Source: CAD feature listing. Evaluate the final solid. Frame: model axes, mm. Coordinates: 2 decimals unless noted, no trailing zeros. Order: outer loops, then holes, each group sorted by start corner. A loop starts at its lowest first (then second) coordinate and runs counter-clockwise, first axis right, second up. Notation, with made-up numbers: (-24, 0) - (15, 0) arc R26 ccw to (15, 26) - close; hole circle Ø6 at (49, -36.75). An arc over 180 degrees is marked (long way). One line per question, with ' | ' between items.
from build123d import *

# Parameters (mm, degrees)
F0_R     = 57.15
F0_R_2   = 9.525
F1_DEPTH = 3.175


with BuildPart() as f1:
    # F0 (on Front) → F1 (new body, symmetric)
    with BuildSketch(Plane.XZ):
        Circle(F0_R)
        with BuildLine():
            ThreePointArc((-32.267608, -44.82798), (-36.315903, -39.658594), (-31.489624, -35.206824))
            ThreePointArc((-31.489624, -35.206824), (-31.099362, -35.222577), (-30.711639, -35.269733))
            ThreePointArc((-30.711639, -35.269733), (-10.931764, -30.012682), (1.53061, -13.777866))
            ThreePointArc((1.53061, -13.777866), (1.553959, -13.706546), (1.578414, -13.635598))
            ThreePointArc((1.578414, -13.635598), (7.66651, -10.668663), (10.727742, -16.709895))
            ThreePointArc((10.727742, -16.709895), (10.704393, -16.781215), (10.679938, -16.852163))
            ThreePointArc((10.679938, -16.852163), (-5.618196, -38.070526), (-31.489624, -44.890889))
            ThreePointArc((-31.489624, -44.890889), (-31.879886, -44.875136), (-32.267608, -44.82798))
        make_face(mode=Mode.SUBTRACT)
        with BuildLine():
            ThreePointArc((-54.514813, -8.881524), (-53.722082, -2.36364), (-47.16151, -2.628457))
            ThreePointArc((-47.16151, -2.628457), (-46.896692, -2.915553), (-46.655876, -3.223059))
            ThreePointArc((-46.655876, -3.223059), (-28.952096, -13.492246), (-8.660118, -10.824727))
            ThreePointArc((-8.660118, -10.824727), (-8.593177, -10.790807), (-8.525717, -10.757931))
            ThreePointArc((-8.525717, -10.757931), (-2.122843, -12.964926), (-4.230021, -19.401339))
            ThreePointArc((-4.230021, -19.401339), (-4.296962, -19.43526), (-4.364422, -19.468135))
            ThreePointArc((-4.364422, -19.468135), (-30.892592, -22.947263), (-54.009178, -9.476126))
            ThreePointArc((-54.009178, -9.476126), (-54.273996, -9.18903), (-54.514813, -8.881524))
        make_face(mode=Mode.SUBTRACT)
        with BuildLine():
            ThreePointArc((8.881524, -54.514813), (2.36364, -53.722082), (2.628457, -47.16151))
            ThreePointArc((2.628457, -47.16151), (2.915553, -46.896692), (3.223059, -46.655876))
            ThreePointArc((3.223059, -46.655876), (13.492246, -28.952096), (10.824727, -8.660118))
            ThreePointArc((10.824727, -8.660118), (10.790807, -8.593177), (10.757931, -8.525717))
            ThreePointArc((10.757931, -8.525717), (12.964926, -2.122843), (19.401339, -4.230021))
            ThreePointArc((19.401339, -4.230021), (19.43526, -4.296962), (19.468135, -4.364422))
            ThreePointArc((19.468135, -4.364422), (22.947263, -30.892592), (9.476126, -54.009178))
            ThreePointArc((9.476126, -54.009178), (9.18903, -54.273996), (8.881524, -54.514813))
        make_face(mode=Mode.SUBTRACT)
        with BuildLine():
            ThreePointArc((44.82798, -32.267608), (39.658594, -36.315903), (35.206824, -31.489624))
            ThreePointArc((35.206824, -31.489624), (35.222577, -31.099362), (35.269733, -30.711639))
            ThreePointArc((35.269733, -30.711639), (30.012682, -10.931764), (13.777866, 1.53061))
            ThreePointArc((13.777866, 1.53061), (13.706546, 1.553959), (13.635598, 1.578414))
            ThreePointArc((13.635598, 1.578414), (10.668663, 7.66651), (16.709895, 10.727742))
            ThreePointArc((16.709895, 10.727742), (16.781215, 10.704393), (16.852163, 10.679938))
            ThreePointArc((16.852163, 10.679938), (38.070526, -5.618196), (44.890889, -31.489624))
            ThreePointArc((44.890889, -31.489624), (44.875136, -31.879886), (44.82798, -32.267608))
        make_face(mode=Mode.SUBTRACT)
        with BuildLine():
            ThreePointArc((-44.82798, 32.267608), (-39.658594, 36.315903), (-35.206824, 31.489624))
            ThreePointArc((-35.206824, 31.489624), (-35.222577, 31.099362), (-35.269733, 30.711639))
            ThreePointArc((-35.269733, 30.711639), (-30.012682, 10.931764), (-13.777866, -1.53061))
            ThreePointArc((-13.777866, -1.53061), (-13.706546, -1.553959), (-13.635598, -1.578414))
            ThreePointArc((-13.635598, -1.578414), (-10.668663, -7.66651), (-16.709895, -10.727742))
            ThreePointArc((-16.709895, -10.727742), (-16.781215, -10.704393), (-16.852163, -10.679938))
            ThreePointArc((-16.852163, -10.679938), (-38.070526, 5.618196), (-44.890889, 31.489624))
            ThreePointArc((-44.890889, 31.489624), (-44.875136, 31.879886), (-44.82798, 32.267608))
        make_face(mode=Mode.SUBTRACT)
        with BuildLine():
            ThreePointArc((-8.881524, 54.514813), (-2.36364, 53.722082), (-2.628457, 47.16151))
            ThreePointArc((-2.628457, 47.16151), (-2.915553, 46.896692), (-3.223059, 46.655876))
            ThreePointArc((-3.223059, 46.655876), (-13.492246, 28.952096), (-10.824727, 8.660118))
            ThreePointArc((-10.824727, 8.660118), (-10.790807, 8.593177), (-10.757931, 8.525717))
            ThreePointArc((-10.757931, 8.525717), (-12.964926, 2.122843), (-19.401339, 4.230021))
            ThreePointArc((-19.401339, 4.230021), (-19.43526, 4.296962), (-19.468135, 4.364422))
            ThreePointArc((-19.468135, 4.364422), (-22.947263, 30.892592), (-9.476126, 54.009178))
            ThreePointArc((-9.476126, 54.009178), (-9.18903, 54.273996), (-8.881524, 54.514813))
        make_face(mode=Mode.SUBTRACT)
        Circle(F0_R_2, mode=Mode.SUBTRACT)
        with BuildLine():
            ThreePointArc((54.514813, 8.881524), (53.722082, 2.36364), (47.16151, 2.628457))
            ThreePointArc((47.16151, 2.628457), (46.896692, 2.915553), (46.655876, 3.223059))
            ThreePointArc((46.655876, 3.223059), (28.952096, 13.492246), (8.660118, 10.824727))
            ThreePointArc((8.660118, 10.824727), (8.593177, 10.790807), (8.525717, 10.757931))
            ThreePointArc((8.525717, 10.757931), (2.122843, 12.964926), (4.230021, 19.401339))
            ThreePointArc((4.230021, 19.401339), (4.296962, 19.43526), (4.364422, 19.468135))
            ThreePointArc((4.364422, 19.468135), (30.892592, 22.947263), (54.009178, 9.476126))
            ThreePointArc((54.009178, 9.476126), (54.273996, 9.18903), (54.514813, 8.881524))
        make_face(mode=Mode.SUBTRACT)
        with BuildLine():
            ThreePointArc((32.267608, 44.82798), (36.315903, 39.658594), (31.489624, 35.206824))
            ThreePointArc((31.489624, 35.206824), (31.099362, 35.222577), (30.711639, 35.269733))
            ThreePointArc((30.711639, 35.269733), (10.931764, 30.012682), (-1.53061, 13.777866))
            ThreePointArc((-1.53061, 13.777866), (-1.553959, 13.706546), (-1.578414, 13.635598))
            ThreePointArc((-1.578414, 13.635598), (-7.66651, 10.668663), (-10.727742, 16.709895))
            ThreePointArc((-10.727742, 16.709895), (-10.704393, 16.781215), (-10.679938, 16.852163))
            ThreePointArc((-10.679938, 16.852163), (5.618196, 38.070526), (31.489624, 44.890889))
            ThreePointArc((31.489624, 44.890889), (31.879886, 44.875136), (32.267608, 44.82798))
        make_face(mode=Mode.SUBTRACT)
    extrude(amount=F1_DEPTH, both=True)


solid = f1.part
(1) Cut plane C-C (z = 49.5). Return the cut outline in (x, y) (3 decimals), and give its area (3 significant figures).
Taken from the geometry:
outline: (-28.563, -3.175) - (-13.937, -3.175) - (-13.937, 3.175) - (-28.563, 3.175) - close; (-1.333, -3.175) - (28.563, -3.175) - (28.563, 3.175) - (-1.333, 3.175) - close | area: 283 mm²
(2) Pull-direction query (X, two-part tool) for faces 1 (the cylindrical face through (5.302, -0.044, 37.858)), 2 (the flat face through (12, 3.175, 1)); classes: pulls with the +X half, pulls with the -X half, needs draft (parallel to the pull), parting line crosses it, or undercut.
Taken from the geometry:
face 1: undercut | face 2: needs draft
(3) Pin query (flat end, axial travel): P1, Ø1.5, axis at y = 1, z = 16, coming from the -X side; P2, Ø1, axis at x = -5, y = -0.5, coming from the +Z side; P3, Ø17, axis at x = 0, z = 0, coming from the +Y side; P4, Ø1, axis at x = -38, y = 0, coming from the +Z side. Return the tip coordinate at first contact, or that it passes through.
Taken from the geometry:
P1: stops at x = -55.08 | P2: stops at z = 56.97 | P3: passes through | P4: stops at z = 43.13
(4) Material intervals for L1, parallel to Z at x = 42, y = 2.5; L2, parallel to Z at x = 2, y = 0.25 (3 decimals); L3, parallel to X at y = 1, z = 17.5, sorted ascending. Write a range as from..to.
Taken from the geometry:
L1: z = -38.76..-35.92, -13.08..7.59, 19..38.76 | L2: z = -57.115..-53.236, -47.935..-31.546, -12.745..-9.313, 9.313..13.232, 16.994..21.018, 35.369..57.115 | L3: x = -54.4..-43.5, -33.36..-23.43, -13.68..-10.45, 0..2.25, 44.62..54.4
(5) Cut plane A-A (z = -28). Return the cut outline in (x, y) (3 decimals), and give its area (3 significant figures).
Taken from the geometry:
outline: (-49.821, -3.175) - (-8.234, -3.175) - (-8.234, 3.175) - (-49.821, 3.175) - close; (4.902, -3.175) - (13.668, -3.175) - (13.668, 3.175) - (4.902, 3.175) - close; (23.424, -3.175) - (35.339, -3.175) - (35.339, 3.175) - (23.424, 3.175) - close; (44.992, -3.175) - (49.821, -3.175) - (49.821, 3.175) - (44.992, 3.175) - close | area: 426 mm²
(6) Cut plane B-B (x = 38.5). Return the cut outline in (y, z) (3 decimals), and give its area (3 significant figures).
Taken from the geometry:
outline: (-3.175, -42.236) - (3.175, -42.236) - (3.175, -36.077) - (-3.175, -36.077) - close; (-3.175, -6.278) - (3.175, -6.278) - (3.175, 9.912) - (-3.175, 9.912) - close; (-3.175, 20.637) - (3.175, 20.637) - (3.175, 42.236) - (-3.175, 42.236) - close | area: 279 mm²
